from build123d import *

# Parameters (mm, degrees)
SKETCH_1_W      = 90
SKETCH_1_H      = 86
SKETCH_1_R      = 1.5
SKETCH_1_R_2    = 2
EXTRUDE_1_DEPTH = 5
FILLET_1_R      = 5


with BuildPart() as part:
    # 草图1 → 凸台-拉伸1 (new body)
    with BuildSketch(Plane(origin=(0, 0, 0), x_dir=(1, 0, 0), z_dir=(0, 1, 0))):
        Rectangle(SKETCH_1_W, SKETCH_1_H)
        with Locations(Location((0, 29.5, 0), (0, 0, 270))):
            Circle(SKETCH_1_R, mode=Mode.SUBTRACT)
        with Locations(Location((20.859650045, 20.859650045, 0), (0, 0, 270))):
            Circle(SKETCH_1_R, mode=Mode.SUBTRACT)
        with Locations(Location((29.5, 0, 0), (0, 0, 270))):
            Circle(SKETCH_1_R, mode=Mode.SUBTRACT)
        with Locations(Location((20.859650045, -20.859650045, 0), (0, 0, 270))):
            Circle(SKETCH_1_R, mode=Mode.SUBTRACT)
        with Locations(Location((0, -29.5, 0), (0, 0, 270))):
            Circle(SKETCH_1_R, mode=Mode.SUBTRACT)
        with Locations(Location((-20.859650045, -20.859650045, 0), (0, 0, 270))):
            Circle(SKETCH_1_R, mode=Mode.SUBTRACT)
        with Locations(Location((-29.5, 0, 0), (0, 0, 270))):
            Circle(SKETCH_1_R, mode=Mode.SUBTRACT)
        with Locations(Location((-20.859650045, 20.859650045, 0), (0, 0, 270))):
            Circle(SKETCH_1_R, mode=Mode.SUBTRACT)
        with Locations(Location((-40, 0, 0), (0, 0, 270))):
            Circle(SKETCH_1_R_2, mode=Mode.SUBTRACT)
        with Locations(Location((40, 0, 0), (0, 0, 90))):
            Circle(SKETCH_1_R_2, mode=Mode.SUBTRACT)
        with Locations(Location((-40, 37, 0), (0, 0, 270))):
            Circle(SKETCH_1_R_2, mode=Mode.SUBTRACT)
        with Locations(Location((40, 37, 0), (0, 0, 90))):
            Circle(SKETCH_1_R_2, mode=Mode.SUBTRACT)
        with Locations(Location((40, -37, 0), (0, 0, 270))):
            Circle(SKETCH_1_R_2, mode=Mode.SUBTRACT)
        with Locations(Location((-40, -37, 0), (0, 0, 90))):
            Circle(SKETCH_1_R_2, mode=Mode.SUBTRACT)
    extrude(amount=EXTRUDE_1_DEPTH)

    # 圆角1
    fillet_1_edges = [part.edges().sort_by_distance(p)[0] for p in [
        (-45, 2.5, -43),
        (45, 2.5, -43),
        (45, 2.5, 43),
        (-45, 2.5, 43),
    ]]
    fillet(fillet_1_edges, radius=FILLET_1_R)


solid = part.part
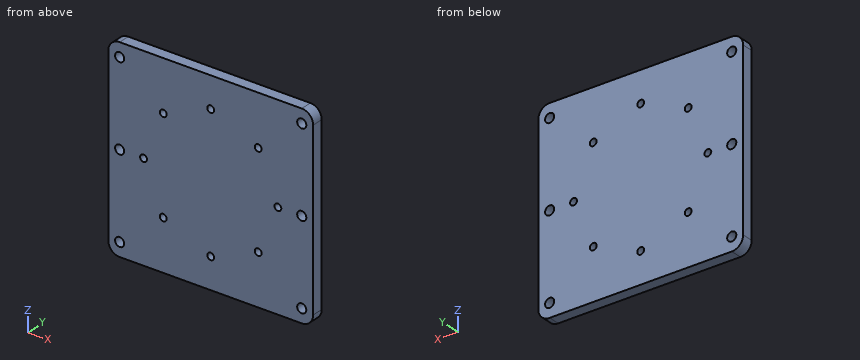
Input: part model. Units: mm. Frame: model coordinates. Give positions to 0.01 mm unless a question says otherwise; leave off trailing zeros. Order: outer loops, then holes, each group sorted by start corner. A loop starts at its lowest first (then second) coordinate and runs counter-clockwise, first axis right, second up.
Q1. Section C-C on x = 0. Output: boundary loops of the cut face in (y, z).
Checked values:
outline: (0, -43) - (5, -43) - (5, -31) - (0, -31) - close; (0, -28) - (5, -28) - (5, 28) - (0, 28) - close; (0, 31) - (5, 31) - (5, 43) - (0, 43) - close
Q2. Section D-D on z = -29.5. Output: boundary loops of the cut face in (x, y), and give its area (3 significant figures).
Checked values:
outline: (-45, 0) - (-1.5, 0) - (-1.5, 5) - (-45, 5) - close; (1.5, 0) - (45, 0) - (45, 5) - (1.5, 5) - close
area: 435 mm2
Q3. Contact query for a flat-ended pin moving along its axis: pin 1 Ø2.5 at (x, z) = (40, 0) entering from -Y. Output: stop coordinate, or through.
Checked values:
pin 1: passes through
Q4. Ray query, probe 1 along X at (y, z) = (1.3, 37); probe 2 along X at (y, z) = (1.9, 0); probe 3 along Z at (x, y) = (-0.5, 4.25). Return the intervals inside material, ascending.
Checked values:
probe 1: x = -45 to -42, -38 to 38, 42 to 45
probe 2: x = -45 to -42, -38 to -31, -28 to 28, 31 to 38, 42 to 45
probe 3: z = -43 to -30.91, -28.09 to 28.09, 30.91 to 43
Q5. Section B-B on z = 37. Output: boundary loops of the cut face in (x, y), and give its area (3 significant figures).
Checked values:
outline: (-45, 0) - (-42, 0) - (-42, 5) - (-45, 5) - close; (-38, 0) - (38, 0) - (38, 5) - (-38, 5) - close; (42, 0) - (45, 0) - (45, 5) - (42, 5) - close
area: 410 mm2
Q6. Section A-A on x = -29.5. Output: boundary loops of the cut face in (y, z).
Checked values:
outline: (0, -43) - (5, -43) - (5, -1.5) - (0, -1.5) - close; (0, 1.5) - (5, 1.5) - (5, 43) - (0, 43) - close
